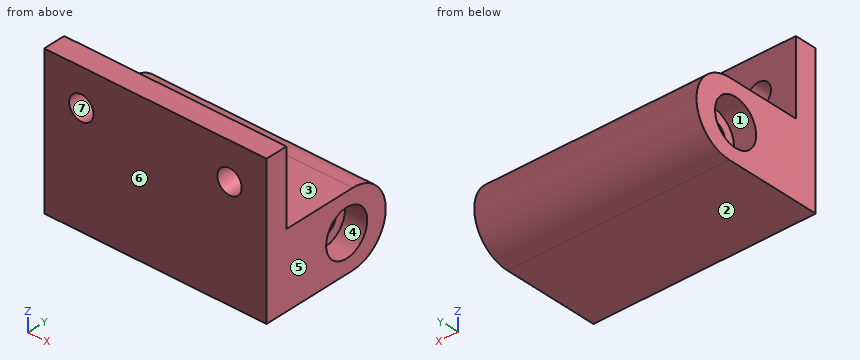
from build123d import *

# Parameters (mm, degrees)
SKETCH1_W           = 30
SKETCH1_H           = 30
BOSS_EXTRUDE1_DEPTH = 22.1
SKETCH2_R           = 3.1
CUT_EXTRUDE1_DEPTH  = 3
SKETCH3_R           = 1.75
CUT_EXTRUDE2_DEPTH  = 38.979073185
CUT_EXTRUDE3_START  = -3
SKETCH4_R           = 3.1
CUT_EXTRUDE3_DEPTH  = 3
SKETCH5_R           = 1.649559613
CUT_EXTRUDE4_DEPTH  = 31.633478418
CUT_EXTRUDE5_DEPTH  = 41.167275237


with BuildPart() as part:
    # Sketch1 → Boss-Extrude1 (new body)
    with BuildSketch(Plane(origin=(0, 0, 0), x_dir=(1, 0, 0), z_dir=(0, 1, 0))):
        Rectangle(SKETCH1_W, SKETCH1_H)
    extrude(amount=BOSS_EXTRUDE1_DEPTH)

    # Sketch2 → Cut-Extrude1 (cut)
    with BuildSketch(Plane(origin=(15, 0, 0), x_dir=(0, 0, -1), z_dir=(1, 0, 0))):
        with Locations((0, 12.1)):
            Circle(SKETCH2_R)
    extrude(amount=-CUT_EXTRUDE1_DEPTH, mode=Mode.SUBTRACT)

    # Sketch3 → Cut-Extrude2 (cut, through all)
    with BuildSketch(Plane(origin=(12, 0, 0), x_dir=(0, 0, -1), z_dir=(1, 0, 0))):
        with Locations((0, 12.1)):
            Circle(SKETCH3_R)
    extrude(amount=-CUT_EXTRUDE2_DEPTH, mode=Mode.SUBTRACT)

    # Sketch4 → Cut-Extrude3 (cut)
    with BuildSketch(Plane.ZY.offset(15).offset(CUT_EXTRUDE3_START)):
        with Locations(Location((0, 12.1, 0), (0, 0, 180))):
            Circle(SKETCH4_R)
    extrude(amount=CUT_EXTRUDE3_DEPTH, mode=Mode.SUBTRACT)

    # Sketch5 → Cut-Extrude4 (cut, through all)
    with BuildSketch(Plane(origin=(0, 22.1, 0), x_dir=(1, 0, 0), z_dir=(0, 1, 0))):
        with Locations(Location((-10, 10, 0), (0, 0, 270))):
            Circle(SKETCH5_R)
        with Locations(Location((10, 10, 0), (0, 0, 270))):
            Circle(SKETCH5_R)
        with Locations(Location((10, -10, 0), (0, 0, 270))):
            Circle(SKETCH5_R)
        with Locations(Location((-10, -10, 0), (0, 0, 270))):
            Circle(SKETCH5_R)
    extrude(amount=-CUT_EXTRUDE4_DEPTH, mode=Mode.SUBTRACT)

    # Sketch6 → Cut-Extrude5 (cut, through all)
    with BuildSketch(Plane.ZY.offset(15)):
        with BuildLine():
            Line((-5, 3), (-5, 13))
            ThreePointArc((-5, 13), (0, 18), (5, 13))
            Line((5, 13), (5, 3))
            Line((5, 3), (15, 3))
            Line((15, 3), (15, 22.1))
            Line((15, 22.1), (-15, 22.1))
            Line((-15, 22.1), (-15, 3))
            Line((-15, 3), (-15, 0))
            Line((-15, 0), (-5, 0))
            Line((-5, 0), (-5, 3))
        make_face()
    extrude(amount=-CUT_EXTRUDE5_DEPTH, mode=Mode.SUBTRACT)


solid = part.part
Geometry check sheet. Reference: the model listing, model coordinates, mm. Face numbers are marked on the shaded views. A direction names the side the tool comes from. Round coordinates to 2 decimals unless told otherwise and drop trailing zeros. Write each loop counter-clockwise with the first axis right and the second up, starting at its lowest first coordinate (ties: lowest second). Pieces come first, ordered by that corner, then holes.
Item 1: Access from +Z, -Z, +X, -X, +Y, -Y to the whole of each face (thin tool, end or side, straight path). Record for the marked faces 1, 2, 3 and 4.
Determined:
face 1: -X
face 2: -Z, +X, -X, +Y, -Y
face 3: +Z, +X, -X, +Y
face 4: +X
Item 2: Section check C-C (z = 10). Record the boundary of the cut face in (x, y), plus the area to 3 significant figures.
Determined:
outline: (-15, 0) - (-11.65, 0) - (-11.65, 3) - (-15, 3) - close; (-8.35, 0) - (8.35, 0) - (8.35, 3) - (-8.35, 3) - close; (11.65, 0) - (15, 0) - (15, 3) - (11.65, 3) - close
area: 70.2 mm2
Item 3: Section check A-A (x = -10). Record the boundary of the cut face in (y, z).
Determined:
outline: (0, -5) - (13, -5) arc R5 ccw to (13, 5) - (3, 5) - (3, 8.35) - (0, 8.35) - close; (0, 11.65) - (3, 11.65) - (3, 15) - (0, 15) - close; hole circle Ø3.5 at (12.1, 0)
Item 4: Go/stop test with flat-tipped pins: pin 1 Ø8 at (x, z) = (-2, 7.5) entering from +Y; pin 2 Ø5 at (y, z) = (12.1, 0) entering from +X; pin 3 Ø1.5 at (x, y) = (10.5, 8.5) entering from +Z; pin 4 Ø8 at (y, z) = (12.1, 0) entering from -X. Record where each tip stops, or that it passes through.
Determined:
pin 1: stops at y = 16.57
pin 2: stops at x = 12
pin 3: stops at z = 5
pin 4: stops at x = -15
Item 5: Material ranges on line 1 along X through (y, z) = (1.1, 10); line 2 along Y through (x, z) = (-13.55, 0); line 3 along Z through (x, y) = (-13.9, 12.1), recorded low to high.
Determined:
line 1: x = -15 to -11.65, -8.35 to 8.35, 11.65 to 15
line 2: y = 0 to 9, 15.2 to 18
line 3: z = -5 to -3.1, 3.1 to 5
Item 6: Section check D-D (x = -5). Record the boundary of the cut face in (y, z).
Determined:
outline: (0, -5) - (13, -5) arc R5 ccw to (13, 5) - (3, 5) - (3, 15) - (0, 15) - close; hole circle Ø3.5 at (12.1, 0)
Item 7: Mould release check, pull along X, two halves, no side actions. Record for the marked faces 5, 6 and 7: +X half, -X half, draft (parallel to the pull), parting line (faces both ways), or undercut.
Determined:
face 5: +X half
face 6: draft
face 7: undercut
Item 8: Section check B-B (y = 12.1). Record the boundary of the cut face in (x, z).
Determined:
outline: (-15, -5) - (15, -5) - (15, -3.1) - (12, -3.1) - (12, -1.75) - (-12, -1.75) - (-12, -3.1) - (-15, -3.1) - close; (-15, 3.1) - (-12, 3.1) - (-12, 1.75) - (12, 1.75) - (12, 3.1) - (15, 3.1) - (15, 5) - (-15, 5) - close
